from build123d import *

# Parameters (mm, degrees)
SKETCH_W        = 123.7
SKETCH_H        = 19.8
PAD_DEPTH       = 3
SKETCH001_W     = 117.7
SKETCH001_H     = 13.8
PAD001_DEPTH    = 16
SKETCH002_R     = 1.85
POCKET_DEPTH    = 18
CHAMFER_SIZE    = 1
SKETCH003_R     = 1.25
POCKET001_DEPTH = 5
CHAMFER001_SIZE = 1
FILLET_R        = 1
CHAMFER002_SIZE = 0.3


with BuildPart() as part:
    # Sketch → Pad (new body)
    with BuildSketch(Plane.XY):
        Rectangle(SKETCH_W, SKETCH_H)
    extrude(amount=PAD_DEPTH)

    # Sketch001 (on Face6 of Pad) → Pad001 (join)
    with BuildSketch(Plane.XY.offset(3)):
        Rectangle(SKETCH001_W, SKETCH001_H)
    extrude(amount=PAD001_DEPTH)

    # Sketch002 (on Face4 of Pad001) → Pocket (cut)
    with BuildSketch(Plane(origin=(0, 0, 0), x_dir=(1, 0, 0), z_dir=(0, 0, -1))):
        with Locations((-45.55, 0)):
            Circle(SKETCH002_R)
        with Locations((-15.55, 0)):
            Circle(SKETCH002_R)
        with Locations((14.45, 0)):
            Circle(SKETCH002_R)
        with Locations((44.45, 0)):
            Circle(SKETCH002_R)
    extrude(amount=-POCKET_DEPTH, mode=Mode.SUBTRACT)

    # Chamfer
    chamfer_edges = [part.edges().sort_by_distance(p)[0] for p in [
        (0, 9.9, 3),
        (-61.85, 0, 3),
        (61.85, 0, 3),
        (0, -9.9, 3),
    ]]
    chamfer(chamfer_edges, length=CHAMFER_SIZE)

    # Sketch003 → Pocket001 (cut)
    with BuildSketch(Plane(origin=(0, 0, 18), x_dir=(1, 0, 0), z_dir=(0, 0, -1))):
        with Locations((-45.55, 0)):
            Circle(SKETCH003_R)
        with Locations((-15.55, 0)):
            Circle(SKETCH003_R)
        with Locations((14.45, 0)):
            Circle(SKETCH003_R)
        with Locations((44.45, 0)):
            Circle(SKETCH003_R)
    extrude(amount=-POCKET001_DEPTH, mode=Mode.SUBTRACT)

    # Chamfer001
    chamfer001_edges = [part.edges().sort_by_distance(p)[0] for p in [
        (0, -6.9, 19),
        (0, 6.9, 19),
        (-58.85, 0, 19),
        (58.85, 0, 19),
    ]]
    chamfer(chamfer001_edges, length=CHAMFER001_SIZE)

    # Fillet
    fillet_edges = [part.edges().sort_by_distance(p)[0] for p in [
        (58.85, -6.9, 10.5),
        (58.85, 6.9, 10.5),
        (61.85, 9.9, 1),
        (61.85, -9.9, 1),
        (-58.85, -6.9, 10.5),
        (-58.85, 6.9, 10.5),
        (-61.85, 9.9, 1),
        (-61.85, -9.9, 1),
    ]]
    fillet(fillet_edges, radius=FILLET_R)

    # Chamfer002
    chamfer002_edges = [part.edges().sort_by_distance(p)[0] for p in [
        (-47.4, 0, 0),
        (-17.4, 0, 0),
        (12.6, 0, 0),
        (42.6, 0, 0),
    ]]
    chamfer(chamfer002_edges, length=CHAMFER002_SIZE)


solid = part.part
CAD build for the part. Positions are in the model's coordinates, mm. A direction names the side the tool comes from. Give positions to 0.01 mm unless a question says otherwise; leave off trailing zeros. Loops run counter-clockwise (first coordinate to the right, second up) from the corner with the lowest first, then second, coordinate; pieces in that order, holes last. Notation, with made-up numbers: M 66,52.5 L 116,52.5 A21 ccw 116,79.5 Z; hole C 66.25,61.25 d11. An arc over 180 degrees is marked long. One line per question, with ' | ' between items. Start each with the question number.
1. Flat gauge pins, fed straight in: pin 1 (6 mm diameter, centred on y = 2, z = 12.5, fed in from -X); pin 2 (1.1 mm diameter, centred on x = -15, y = 0.5, fed in from -Z); pin 3 (9.5 mm diameter, centred on y = -1, z = 9, fed in from +X). Where does each tip first touch, or does it go through?
2. Saw through at D-D on y = 0. State how many separate pieces and enclosed holes the cut face has, plus the area to 3 significant figures.
3. Saw through at A-A on z = 9.25. Give the cut face in (x, y).
4. Probe L1, parallel to X at y = 0, z = 9.25; L2, parallel to Y at x = 44.45, z = 9.5; L3, parallel to Y at x = -38.5, z = 8.5. List the from-to ranges inside material, lowest first. Write a range as from..to.
5. Two-plate mould, pull along Y, no slides. Class faces 6 (the face through (58.85, 0, 10)), 7 (the face through (43.2, -0.05, 18.49)), 8 (the face through (-44, 0, 18)), 9 (the face through (-1, -6.9, 10)): pulls with the +Y half, pulls with the -Y half, needs draft (parallel to the pull), parting line crosses it, or undercut.
6. 3-axis set-ups, long thin cutter, end or side, ignore diameter. For faces 1 (the face through (-1, -9.9, 1)), 2 (the face through (-58.85, 0, 10)), 3 (the face through (-1, 6.9, 10)), 4 (the face through (-61.85, 0, 1)), 5 (the face through (46, 0, 18)): which of +Z, -Z, +X, -X, +Y, -Y reach the whole face in a straight line?
7. Saw through at C-C on x = 20. Give the cut face in (y, z), plus the area to 3 significant figures.
8. Saw through at B-B on x = -45.55. Give the cut face in (y, z).
Result sheet:
1) pin 1: stops at x = -58.85 | pin 2: stops at z = 18 | pin 3: stops at x = 58.85
2) separate pieces: 5 | enclosed holes: 0 | area: 1,980 mm^2
3) outline: M -58.85,-5.9 A1 ccw -57.85,-6.9 L 57.85,-6.9 A1 ccw 58.85,-5.9 L 58.85,5.9 A1 ccw 57.85,6.9 L -57.85,6.9 A1 ccw -58.85,5.9 Z; hole C -45.55,0 d3.7; hole C -15.55,0 d3.7; hole C 14.45,0 d3.7; hole C 44.45,0 d3.7
4) L1: x = -58.85..-47.4, -43.7..-17.4, -13.7..12.6, 16.3..42.6, 46.3..58.85 | L2: y = -6.9..-1.85, 1.85..6.9 | L3: y = -6.9..6.9
5) face 6: needs draft | face 7: undercut | face 8: undercut | face 9: pulls with the -Y half
6) face 1: +Z, -Z, +X, -X, -Y | face 2: +Z, -X, +Y, -Y | face 3: +Z, +X, -X, +Y | face 4: +Z, -Z, -X, +Y, -Y | face 5: -Z
7) outline: M -9.9,0 L 9.9,0 L 9.9,2 L 8.9,3 L 6.9,3 L 6.9,18 L 5.9,19 L -5.9,19 L -6.9,18 L -6.9,3 L -8.9,3 L -9.9,2 Z | area: 278 mm^2
8) outline: M -9.9,0 L -2.15,0 L -1.85,0.3 L -1.85,18 L -1.25,18 L -1.25,19 L -5.9,19 L -6.9,18 L -6.9,3 L -8.9,3 L -9.9,2 Z; M 1.25,18 L 1.85,18 L 1.85,0.3 L 2.15,0 L 9.9,0 L 9.9,2 L 8.9,3 L 6.9,3 L 6.9,18 L 5.9,19 L 1.25,19 Z
